from build123d import *

# Parameters (mm, degrees)
SKETCH_1_W          = 110
SKETCH_1_H          = 140
EXTRUDE_1_DEPTH     = 3
SKETCH_2_R          = 3
CUT_EXTRUDE_1_DEPTH = 3
FILLET_1_R          = 3


with BuildPart() as part:
    # 草图1 → 凸台-拉伸1 (new body)
    with BuildSketch(Plane(origin=(0, 0, 0), x_dir=(1, 0, 0), z_dir=(0, 1, 0))):
        Rectangle(SKETCH_1_W, SKETCH_1_H)
    extrude(amount=EXTRUDE_1_DEPTH)

    # 草图2 → 切除-拉伸1 (cut)
    with BuildSketch(Plane.XZ):
        with Locations(Location((-25, 55, 0), (0, 0, 270))):
            Circle(SKETCH_2_R)
        with Locations(Location((25, 55, 0), (0, 0, 90))):
            Circle(SKETCH_2_R)
    extrude(amount=-CUT_EXTRUDE_1_DEPTH, mode=Mode.SUBTRACT)

    # 圆角1
    fillet_1_edges = [part.edges().sort_by_distance(p)[0] for p in [
        (55, 1.5, 70),
        (-55, 1.5, 70),
        (-55, 1.5, -70),
        (55, 1.5, -70),
    ]]
    fillet(fillet_1_edges, radius=FILLET_1_R)


solid = part.part
For this review, take the finished solid that the model builds, in its own axes (mm). Round coordinates to 2 decimals unless told otherwise and drop trailing zeros. Write each loop counter-clockwise with the first axis right and the second up, starting at its lowest first coordinate (ties: lowest second). Pieces come first, ordered by that corner, then holes. Notation, with made-up numbers: (25, -17.75) - (39, -17.75) arc R26 ccw to (39, 15.25) - close; hole circle Ø5 at (63, -24). An arc over 180 degrees is marked (long way). Use a Markdown table: item, result.
Q1. Wall thickness on line 1 along X through (y, z) = (0.7, 55); line 2 along Z through (x, y) = (25, 1.6): over which ranges is each line inside the solid? List them lowest first.
Derived:
| item | result |
|---|---|
| line 1 | x = -55 to -28, -22 to 22, 28 to 55 |
| line 2 | z = -70 to 52, 58 to 70 |
Q2. We need section B-B (z = 55). Give the boundary of the cut face in (x, y), plus the area to 3 significant figures.
Derived:
| item | result |
|---|---|
| outline | (-55, 0) - (-28, 0) - (-28, 3) - (-55, 3) - close; (-22, 0) - (22, 0) - (22, 3) - (-22, 3) - close; (28, 0) - (55, 0) - (55, 3) - (28, 3) - close |
| area | 294 mm2 |
Q3. The part is to be moulded in two halves that separate along Z. For faces 1 (the cylindrical face through (-25, 1, 58)), 2 (the cylindrical face through (54.1, 1.52, -69.14)), 3 (the cylindrical face through (25, 1, 52)), 4 (the flat face through (-1, 3, -1)), say which applies: pulls with the +Z half, pulls with the -Z half, needs draft (parallel to the pull), parting line crosses it, or undercut.
Derived:
| item | result |
|---|---|
| face 1 | undercut |
| face 2 | pulls with the -Z half |
| face 3 | undercut |
| face 4 | needs draft |
Q4. We need section A-A (x = -25). Give the boundary of the cut face in (y, z), plus the area to 3 significant figures.
Derived:
| item | result |
|---|---|
| outline | (0, -70) - (3, -70) - (3, 52) - (0, 52) - close; (0, 58) - (3, 58) - (3, 70) - (0, 70) - close |
| area | 402 mm2 |
